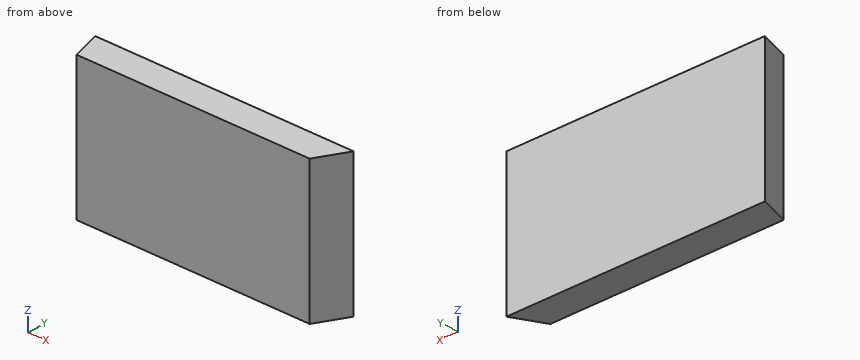
```python
from build123d import *

# Parameters (mm, degrees)
F0_W     = 163.938712
F0_H     = 88.9
F1_DEPTH = 19.05
F3_DEPTH = 88.901
F4_DEPTH = 88.901


with BuildPart() as f1:
    # F0 (on Front) → F1 (new body)
    with BuildSketch(Plane.XZ):
        with Locations((-1133.26766, -1068.65232)):
            Rectangle(F0_W, F0_H)
    extrude(amount=F1_DEPTH)

    # F2 (on face) → F3 (cut, through all)
    with BuildSketch(Plane.XY.offset(-1024.20232)):
        Polygon((-1209.678422, -19.05), (-1215.237016, 0), (-1215.237016, -19.05), align=None)
    extrude(amount=-F3_DEPTH, mode=Mode.SUBTRACT)

    # F2 (on face) → F4 (cut, through all)
    with BuildSketch(Plane.XY.offset(-1024.20232)):
        Polygon((-1051.298304, -19.05), (-1051.298304, 0), (-1061.742284, -19.05), align=None)
    extrude(amount=-F4_DEPTH, mode=Mode.SUBTRACT)


solid = f1.part
```
Could you check a few things on this model? Use its own coordinates, in mm. Coordinates: 2 decimals unless noted, no trailing zeros. Loops run counter-clockwise (first coordinate to the right, second up) from the corner with the lowest first, then second, coordinate; pieces in that order, holes last. Notation, with made-up numbers: M 14.5,51.25 L 65.5,51.25 A14 ccw 65.5,66.25 Z; hole C 19.5,60.25 d10. An arc over 180 degrees is marked long. Put each result on its own line as item: value. Start each with the question number.
(1) Suppose I cut it at A-A on z = -1085. Please give me the cut outline in (x, y), then the cut area to 3 significant figures.
(2) Will these pins go through, and if not, where does the flat tip stop? P1, Ø4, axis at y = -16.5, z = -1103.5, coming from the -X side; P2, Ø5, axis at y = -7.5, z = -1087, coming from the -X side; P3, Ø10, axis at y = -10.5, z = -1075.5, coming from the -X side.
(3) I need wall thicknesses on line 1 (X direction, y = -8.5, z = -1070.5); line 2 (X direction, y = -5.75, z = -1041). Which ranges of each line are inside material? Lowest first, please. Write a range as from..to.
(4) Suppose I cut it at B-B on y = -6.75. Please give me the cut outline in (x, z), then the cut area to 3 significant figures.
Solutions:
1. outline: M -1215.24,0 L -1209.68,-19.05 L -1061.74,-19.05 L -1051.3,0 Z
1. area: 2,970 mm2
2. P1: stops at x = -1211.01
2. P2: stops at x = -1213.78
2. P3: stops at x = -1213.63
3. line 1: x = -1212.76..-1055.96
3. line 2: x = -1213.56..-1054.45
4. outline: M -1213.27,-1113.1 L -1055,-1113.1 L -1055,-1024.2 L -1213.27,-1024.2 Z
4. area: 14,100 mm2
